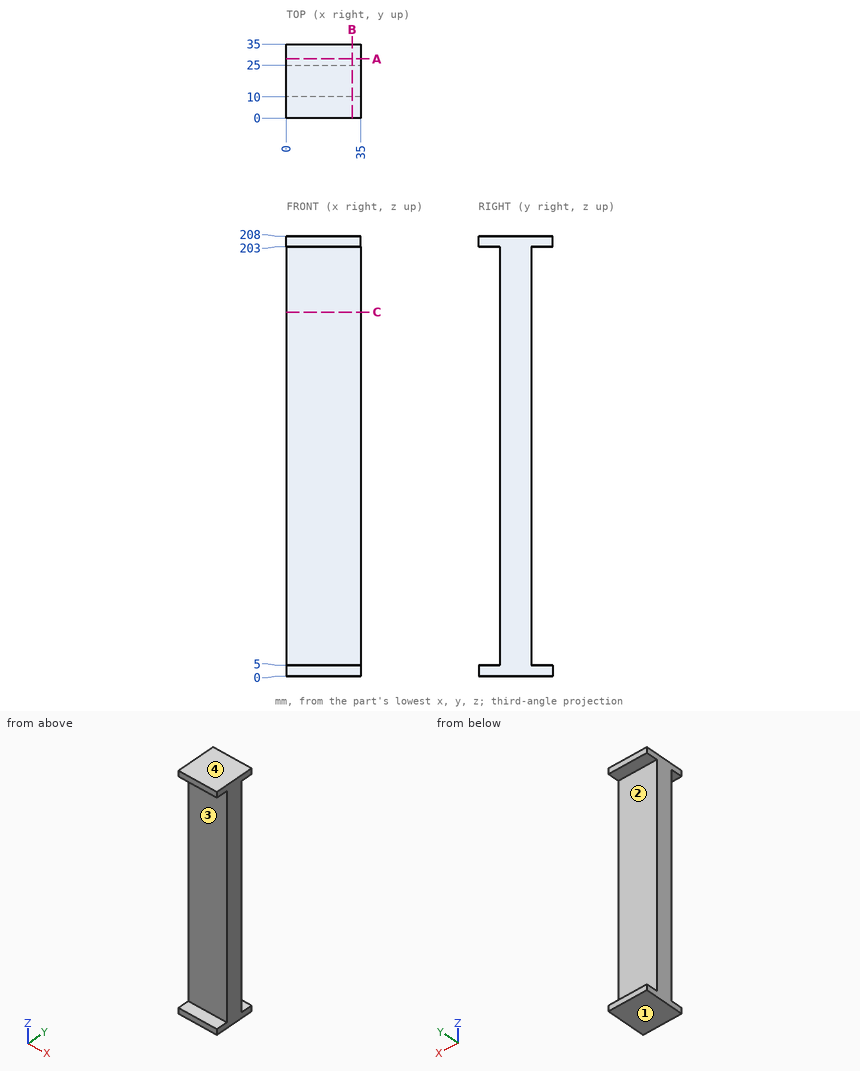
Answer from the drawing. Dimensions are ordinates in mm from the lowest x, y and z of the part. Give positions to 0.01 mm unless a question says otherwise; leave off trailing zeros. Write each loop counter-clockwise with the first axis right and the second up, starting at its lowest first coordinate (ties: lowest second). Pieces come first, ordered by that corner, then holes. Notation, with made-up numbers: (19, 20) - (48, 20) arc R24 cw to (48, 31) - close; hole circle Ø1 at (48.5, 30). An arc over 180 degrees is marked (long way). Answer in a Markdown table with one row per item. Add a question column.
Item 1: Section C-C, the plane z = 172 is taken. Write down the section's boundary in (x, y).
Item 2: Find the intervals of material crossed by L1, parallel to Z at x = 12, y = 9.5; L2, parallel to Y at x = 22, z = 139, in increasing order.
Item 3: Determine the mould class of the marked faces 1, 2, 3 and 4 for opening direction Z: pulls with the +Z half, pulls with the -Z half, needs draft (parallel to the pull), parting line crosses it, or undercut.
Item 4: Section B-B, the plane x = 31 is taken. Write down the section's boundary in (y, z).
Item 5: Section A-A, the plane y = 28 is taken. Write down the section's boundary in (x, z), and give its area (3 significant figures).
Item 6: Flat-ended cylindrical pins translate along their axes: P1, Ø17.5, axis at x = 23.5, z = 71, coming from the -Y side; P2, Ø1.5, axis at x = 10.5, z = 149.5, coming from the +Y side. Find the tip coordinate at first contact, or state that the pin passes through.
Recorded:
| question | item | result |
|---|---|---|
| 1 | outline | (0, 10) - (35, 10) - (35, 25) - (0, 25) - close |
| 2 | L1 | z = 0 to 5, 203 to 208 |
| 2 | L2 | y = 10 to 25 |
| 3 | face 1 | pulls with the -Z half |
| 3 | face 2 | undercut |
| 3 | face 3 | undercut |
| 3 | face 4 | pulls with the +Z half |
| 4 | outline | (0, 0) - (35, 0) - (35, 5) - (25, 5) - (25, 203) - (35, 203) - (35, 208) - (0, 208) - (0, 203) - (10, 203) - (10, 5) - (0, 5) - close |
| 5 | outline | (0, 0) - (35, 0) - (35, 5) - (0, 5) - close; (0, 203) - (35, 203) - (35, 208) - (0, 208) - close |
| 5 | area | 350 mm2 |
| 6 | P1 | stops at y = 10 |
| 6 | P2 | stops at y = 25 |
